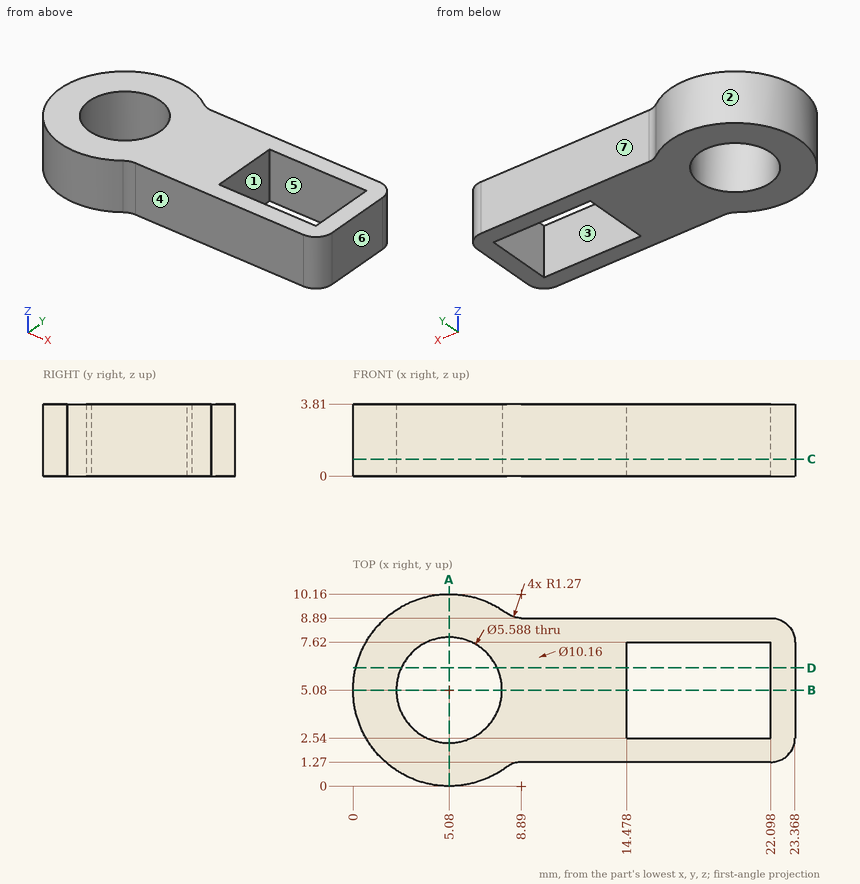
Can you work these out from the drawing? Everything is in mm from the part's minimum corner. A direction names the side the tool comes from. Give positions to 0.01 mm unless a question says otherwise; leave off trailing zeros. Loops run counter-clockwise (first coordinate to the right, second up) from the corner with the lowest first, then second, coordinate; pieces in that order, holes last. Notation, with made-up numbers: (28.5, 17.5) -> (42.5, 17.5) arc R23 ccw to (42.5, 27.5) -> close; hole circle Ø11 at (26.5, 24). An arc over 180 degrees is marked (long way). Put each result on its own line as item: value.
(1) Imagine slicing it at B-B on y = 5.08. Write out the boundary of the cut face in (x, z), plus the area to 3 significant figures.
Computed:
outline: (0, 0) -> (2.29, 0) -> (2.29, 3.81) -> (0, 3.81) -> close; (7.87, 0) -> (14.48, 0) -> (14.48, 3.81) -> (7.87, 3.81) -> close; (22.1, 0) -> (23.37, 0) -> (23.37, 3.81) -> (22.1, 3.81) -> close
area: 38.7 mm^2
(2) Imagine slicing it at A-A on x = 5.08. Write out the boundary of the cut face in (y, z), plus the area to 3 significant figures.
Computed:
outline: (0, 0) -> (2.29, 0) -> (2.29, 3.81) -> (0, 3.81) -> close; (7.87, 0) -> (10.16, 0) -> (10.16, 3.81) -> (7.87, 3.81) -> close
area: 17.4 mm^2
(3) Thinking about a two-plate mould opening in Y: for the marked faces 1, 2, 3 and 4, which applies, pulls with the +Y half, pulls with the -Y half, needs draft (parallel to the pull), parting line crosses it, or undercut?
Computed:
face 1: undercut
face 2: parting line crosses it
face 3: undercut
face 4: pulls with the -Y half
(4) I'm going to push flat-ended pins straight in: pin 1 Ø2 at (y, z) = (1.5, 3) entering from -X; pin 2 Ø3.5 at (x, y) = (5.08, 5.08) entering from +Z; pin 3 Ø1.1 at (x, z) = (18.5, 2.5) entering from +Y; pin 4 Ø1.1 at (x, z) = (18.5, 2) entering from -Y. Where does each tip first touch, or does it pass through?
Computed:
pin 1: x = 0.7
pin 2: through
pin 3: y = 8.89
pin 4: y = 1.27
(5) Please list where these lines run through material, in increasing order: probe 1 along X at (y, z) = (5.08, 1.35); probe 2 along X at (y, z) = (4.25, 2.75); probe 3 along Y at (x, z) = (5.08, 1.05). Write a range as [from, to].
Computed:
probe 1: [0, 2.29], [7.87, 14.48], [22.1, 23.37]
probe 2: [0.07, 2.41], [7.75, 14.48], [22.1, 23.37]
probe 3: [0, 2.29], [7.87, 10.16]
(6) Imagine slicing it at D-D on y = 6.25. Write out the boundary of the cut face in (x, z), plus the area to 3 significant figures.
Computed:
outline: (0.14, 0) -> (2.54, 0) -> (2.54, 3.81) -> (0.14, 3.81) -> close; (7.62, 0) -> (14.48, 0) -> (14.48, 3.81) -> (7.62, 3.81) -> close; (22.1, 0) -> (23.37, 0) -> (23.37, 3.81) -> (22.1, 3.81) -> close
area: 40.1 mm^2
(7) For the marked faces 5, 6 and 7, which set-ups out of +Z, -Z, +X, -X, +Y, -Y let a thin tool reach every point of the face, with its end or its side?
Computed:
face 5: +Z, -Z
face 6: +Z, -Z, +X, +Y, -Y
face 7: +Z, -Z, +X, +Y
(8) Imagine slicing it at C-C on z = 0.9. Write out the boundary of the cut face in (x, y).
Computed:
outline: (8.13, 1.02) arc R1.27 cw to (8.89, 1.27) -> (22.1, 1.27) arc R1.27 ccw to (23.37, 2.54) -> (23.37, 7.62) arc R1.27 ccw to (22.1, 8.89) -> (8.89, 8.89) arc R1.27 cw to (8.13, 9.14) arc R5.08 ccw (long way) to start; hole circle Ø5.59 at (5.08, 5.08); hole (14.48, 2.54) -> (22.1, 2.54) -> (22.1, 7.62) -> (14.48, 7.62) -> close
